```python
from build123d import *

# Parameters (mm, degrees)
BOSS_EXTRUDE1_DEPTH = 6.35
SKETCH2_R           = 2.35
SKETCH2_R_2         = 2.4
SKETCH2_R_3         = 2.325
SKETCH2_R_4         = 2.275
SKETCH2_R_5         = 2.375
SKETCH2_R_6         = 2.425
SKETCH2_R_7         = 2.3
SKETCH2_R_8         = 2.25
SKETCH2_R_9         = 2.225
SKETCH2_R_10        = 2.2
SKETCH2_R_11        = 2.45
SKETCH2_R_12        = 2.475
SKETCH2_R_13        = 2.5
SKETCH2_R_14        = 2.675
SKETCH2_R_15        = 2.7
SKETCH2_W           = 0.929848637
SKETCH2_H           = 0.929848637
CUT_EXTRUDE1_DEPTH  = 6.35


with BuildPart() as part:
    # Sketch1 → Boss-Extrude1 (new body)
    with BuildSketch(Plane(origin=(0, 0, 0), x_dir=(1, 0, 0), z_dir=(0, 1, 0))):
        with BuildLine():
            Line((3, 0), (27, 0))
            ThreePointArc((27, 0), (29.121320344, 0.878679656), (30, 3))
            Line((30, 3), (30, 27))
            ThreePointArc((30, 27), (29.121320344, 29.121320344), (27, 30))
            Line((27, 30), (3, 30))
            ThreePointArc((3, 30), (0.878679656, 29.121320344), (0, 27))
            Line((0, 27), (0, 3))
            ThreePointArc((0, 3), (0.878679656, 0.878679656), (3, 0))
        make_face()
    extrude(amount=BOSS_EXTRUDE1_DEPTH)

    # Sketch2 → Cut-Extrude1 (cut)
    with BuildSketch(Plane(origin=(0, 6.35, 0), x_dir=(1, 0, 0), z_dir=(0, 1, 0))):
        with Locations(Location((4.130390075, 25.933737418, 0), (0, 0, 270))):
            Circle(SKETCH2_R)
        with Locations(Location((17.084143496, 25.933737418, 0), (0, 0, 270))):
            Circle(SKETCH2_R_2)
        with Locations(Location((4.130390075, 18.911777023, 0), (0, 0, 270))):
            Circle(SKETCH2_R_3)
        with Locations(Location((17.084143496, 18.911777023, 0), (0, 0, 270))):
            Circle(SKETCH2_R_4)
        with Locations(Location((10.607266785, 25.933737418, 0), (0, 0, 270))):
            Circle(SKETCH2_R_5)
        with Locations(Location((23.593083953, 25.933737418, 0), (0, 0, 270))):
            Circle(SKETCH2_R_6)
        with Locations(Location((10.863776754, 18.911777023, 0), (0, 0, 270))):
            Circle(SKETCH2_R_7)
        with Locations(Location((23.593083953, 18.911777023, 0), (0, 0, 270))):
            Circle(SKETCH2_R_8)
        with Locations(Location((4.130390075, 12.499027805, 0), (0, 0, 270))):
            Circle(SKETCH2_R_9)
        with Locations(Location((10.607266785, 12.499027805, 0), (0, 0, 270))):
            Circle(SKETCH2_R_10)
        with Locations(Location((17.084143496, 12.499027805, 0), (0, 0, 270))):
            Circle(SKETCH2_R_11)
        with Locations(Location((23.593083953, 12.499027805, 0), (0, 0, 270))):
            Circle(SKETCH2_R_12)
        with Locations(Location((3.938007598, 5.092302457, 0), (0, 0, 270))):
            Circle(SKETCH2_R_13)
        with Locations(Location((10.607266785, 5.092302457, 0), (0, 0, 270))):
            Circle(SKETCH2_R_14)
        with Locations(Location((17.084143496, 5.092302457, 0), (0, 0, 270))):
            Circle(SKETCH2_R_15)
        with Locations(Location((23.593083953, 5.092302457, 0), (0, 0, 270))):
            Circle(SKETCH2_R_3)
        with Locations((27.937721549, 8.218517702)):
            Rectangle(SKETCH2_W, SKETCH2_H)
    extrude(amount=-CUT_EXTRUDE1_DEPTH, mode=Mode.SUBTRACT)


solid = part.part
```
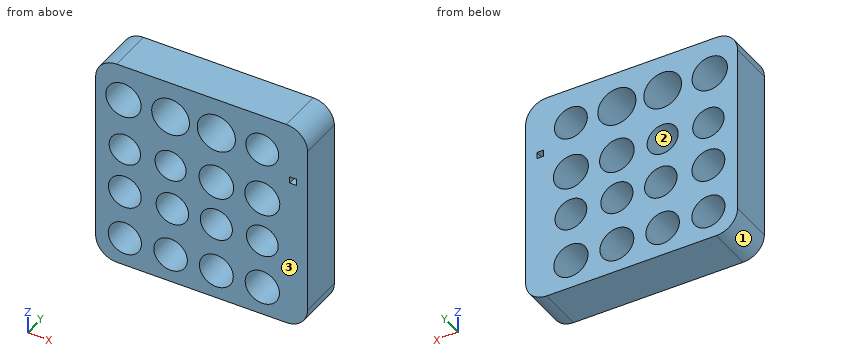
Input: part model. Units: mm. Frame: model coordinates. Face numbers are marked on the shaded views. Round coordinates to 2 decimals unless told otherwise and drop trailing zeros. Loops run counter-clockwise (first coordinate to the right, second up) from the corner with the lowest first, then second, coordinate; pieces in that order, holes last. Notation, with made-up numbers: (59, 37) -> (102, 37) arc R17 ccw to (102, 54) -> close; hole circle Ø8 at (-4.5, 63). An arc over 180 degrees is marked (long way). Use one line per item in the form item = value. Start each with the question number.
Item 1: Section query C-C on y = 1.5. Count the separate pieces of the cut face and the enclosed holes in it, then the cut area to 3 significant figures.
Item 2: Section query A-A on x = 4.75. Return the cut outline in (y, z), then the cut area to 3 significant figures.
Item 3: Contact query for flat-ended pins moving along their axis: pin 1 Ø4.5 at (x, z) = (10.61, -25.93) entering from +Y; pin 2 Ø0.7 at (x, y) = (28, 4) entering from +Z. Output: stop coordinate, or through.
Item 4: Mould query, pull axis Z, two halves, no side actions, for the marked faces 1, 2 and 3. Classes: pulls with the +Z half, pulls with the -Z half, needs draft (parallel to the pull), parting line crosses it, or undercut.
Item 5: Section query B-B on z = -19.5. Return the cut outline in (x, y).
Item 6: Material intervals for L1, parallel to X at y = 1.75, z = -4; L2, parallel to X at y = 4, z = -6; L3, parallel to Z at x = 19, y = 2, sorted ascending. Write a range as from..to.
Ans:
q1.separate_pieces = 1
q1.enclosed_holes = 17
q1.area = 603 mm^2
q2.outline = (0, -30) -> (6.35, -30) -> (6.35, -28.2) -> (0, -28.2) -> close; (0, -23.67) -> (6.35, -23.67) -> (6.35, -21.15) -> (0, -21.15) -> close; (0, -16.67) -> (6.35, -16.67) -> (6.35, -14.64) -> (0, -14.64) -> close; (0, -10.36) -> (6.35, -10.36) -> (6.35, -7.46) -> (0, -7.46) -> close; (0, -2.73) -> (6.35, -2.73) -> (6.35, 0) -> (0, 0) -> close
q2.area = 76.1 mm^2
q3.pin_1 = through
q3.pin_2 = -0.07
q4.face_1 = pulls with the -Z half
q4.face_2 = undercut
q4.face_3 = needs draft
q5.outline = (0, 0) -> (1.88, 0) -> (1.88, 6.35) -> (0, 6.35) -> close; (6.38, 0) -> (8.64, 0) -> (8.64, 6.35) -> (6.38, 6.35) -> close; (13.09, 0) -> (14.89, 0) -> (14.89, 6.35) -> (13.09, 6.35) -> close; (19.28, 0) -> (21.42, 0) -> (21.42, 6.35) -> (19.28, 6.35) -> close; (25.76, 0) -> (30, 0) -> (30, 6.35) -> (25.76, 6.35) -> close
q6.L1 = 0..1.69, 6.19..8.17, 13.05..14.61, 19.55..21.54, 25.65..30
q6.L2 = 0..1.61, 6.27..8.09, 13.12..14.54, 19.63..21.45, 25.73..30
q6.L3 = -30..-27.38, -24.49..-20.14, -17.68..-14.03, -10.97..-6.99, -3.19..0
